Verification items for the finished model (mm, model axes). A direction names the side the tool comes from. Round coordinates to 2 decimals unless told otherwise and drop trailing zeros. Order: outer loops, then holes, each group sorted by start corner. A loop starts at its lowest first (then second) coordinate and runs counter-clockwise, first axis right, second up. Notation, with made-up numbers: (30, 46) -> (88, 46) arc R21 ccw to (88, 60) -> close; hole circle Ø8 at (-9.75, 41). An arc over 180 degrees is marked (long way). Put each result on its own line as item: value.
```python
from build123d import *

# Parameters (mm, degrees)
CROQUIS1_R              = 5.000000001
CROQUIS1_W              = 11.000000002
CROQUIS1_H              = 6.000000001
CROQUIS1_W_2            = 11.000000001
CROQUIS1_W_3            = 83.00000001
CROQUIS1_H_2            = 54.000000007
SALIENTE_EXTRUIR1_DEPTH = 1.5
CROQUIS3_W              = 3
CROQUIS3_H              = 143.999988457
SALIENTE_EXTRUIR2_DEPTH = 15
CROQUIS4_R              = 4.1
CORTAR_EXTRUIR1_DEPTH   = 23
CROQUIS8_W              = 20.699997559
CROQUIS8_H              = 3
SALIENTE_EXTRUIR4_DEPTH = 3
CROQUIS9_W              = 20.699997559
CROQUIS9_H              = 3
SALIENTE_EXTRUIR5_DEPTH = 3


with BuildPart() as part:
    # Croquis1 → Saliente-Extruir1 (new, symmetric)
    with BuildSketch(Plane.XY):
        Polygon((18.699888738, 146.999988499), (-0.000108821, 146.999988499), (-0.000108821, 3.000000042), (18.699888738, 3.000000042), (18.699888738, -1.1561e-05), (31.299897882, -1.1561e-05), (31.299897882, 2.999988439), (39.849897883, 2.999988439), (39.849897883, 6.5452e-05), (48.799897884, 6.5452e-05), (48.799897884, 3.000065452), (51.579549154, 3.000065452), (51.579549154, 6.749716476), (49.079130382, 6.749716476), (49.079130382, 9.750065453), (51.579549154, 9.750065453), (51.579549154, 10.725065453), (54.579549155, 10.725065453), (54.579549155, 9.750065453), (57.079549155, 9.750065453), (57.079549155, 6.749716476), (54.579549155, 6.749716476), (54.579549155, 3.000065452), (57.359200426, 3.000065452), (57.359200426, 9.8389e-05), (66.309200426, 9.8389e-05), (66.309200426, 3.00009839), (74.840541181, 3.00009839), (74.840541181, 9.8305e-05), (87.461202556, 0.000103657), (87.461202556, 3.000103699), (99.999885723, 3.000103699), (99.999885723, 9.999884868), (96.999885722, 9.999884868), (96.999885722, 19.999884869), (99.999885723, 19.999884869), (99.999885723, 29.99988487), (96.999885722, 29.99988487), (96.999885722, 43.437175485), (93.250234699, 43.437175485), (93.250234699, 40.937175485), (90.249885721, 40.937175485), (90.249885721, 43.437175485), (89.274885721, 43.437175485), (89.274885721, 46.437175486), (90.249885721, 46.437175486), (90.249885721, 48.937594258), (93.250234699, 48.937594258), (93.250234699, 46.437175486), (96.999885722, 46.437175486), (96.999885722, 59.874884873), (99.999885723, 59.874884873), (99.999885723, 69.999884875), (96.999885722, 69.999884875), (96.999885722, 79.999884876), (99.999885723, 79.999884876), (99.999885723, 90.124884877), (96.999885722, 90.124884877), (96.999885722, 103.562175492), (93.250234699, 103.562175492), (93.250234699, 101.062175492), (90.249885721, 101.062175492), (90.249885721, 103.562175492), (89.274885721, 103.562175492), (89.274885721, 106.562175493), (90.249885721, 106.562175493), (90.249885721, 109.062594265), (93.250234699, 109.062594265), (93.250234699, 106.562175493), (96.999885722, 106.562175493), (96.999885722, 119.99988488), (99.999885723, 119.99988488), (99.999885723, 129.999884881), (96.999885722, 129.999884881), (96.999885722, 139.999884883), (99.999885723, 139.999884883), (99.999885723, 146.999884842), (87.461202556, 146.999884842), (87.461202556, 149.999884884), (74.840541181, 149.999890236), (74.840541181, 146.999890151), (66.309200426, 146.999890151), (66.309200426, 149.999890151), (57.359200426, 149.999890151), (57.359200426, 146.999923088), (54.579549155, 146.999923088), (54.579549155, 143.250272065), (57.079549155, 143.250272065), (57.079549155, 140.249923087), (54.579549155, 140.249923087), (54.579549155, 139.274923087), (51.579549154, 139.274923087), (51.579549154, 140.249923087), (49.079130382, 140.249923087), (49.079130382, 143.250272065), (51.579549154, 143.250272065), (51.579549154, 146.999923088), (48.799897884, 146.999923088), (48.799897884, 149.999923089), (39.849897883, 149.999923089), (39.849897883, 147.000000101), (31.299897882, 147.000000101), (31.299897882, 150.000000101), (18.699888738, 150.000000101), align=None)
        with Locations((18.167765659, 72.011021453)):
            Circle(CROQUIS1_R, mode=Mode.SUBTRACT)
        with Locations((35.451849713, 72.011021453)):
            Rectangle(CROQUIS1_W, CROQUIS1_H, mode=Mode.SUBTRACT)
        with BuildLine():
            Line((82.774554778, 63.495021452), (82.774554778, 61.971021451))
            Line((82.774554778, 61.971021451), (85.314554779, 59.431021451))
            Line((85.314554779, 59.431021451), (85.314554779, 26.411021447))
            Line((85.314554779, 26.411021447), (82.774554778, 23.871021447))
            Line((82.774554778, 23.871021447), (82.774554778, 12.441021446))
            Line((82.774554778, 12.441021446), (81.504554778, 11.171021446))
            Line((81.504554778, 11.171021446), (17.750554771, 11.171021446))
            ThreePointArc((17.750554771, 11.171021446), (17.032134281, 11.468600956), (16.734554771, 12.187021446))
            Line((16.734554771, 12.187021446), (16.734554771, 63.495021452))
            ThreePointArc((16.734554771, 63.495021452), (17.032134281, 64.213441941), (17.750554771, 64.511021452))
            Line((17.750554771, 64.511021452), (81.758554778, 64.511021452))
            ThreePointArc((81.758554778, 64.511021452), (82.476975268, 64.213441941), (82.774554778, 63.495021452))
        make_face(mode=Mode.SUBTRACT)
        with Locations((57.631849716, 72.011021453)):
            Rectangle(CROQUIS1_W_2, CROQUIS1_H, mode=Mode.SUBTRACT)
        with Locations((79.814554778, 72.011021453)):
            Rectangle(CROQUIS1_W, CROQUIS1_H, mode=Mode.SUBTRACT)
        with Locations((45.799885716, 106.511021457)):
            Rectangle(CROQUIS1_W_3, CROQUIS1_H_2, mode=Mode.SUBTRACT)
        with Locations((15.358852485, 137.999884882)):
            Rectangle(CROQUIS1_W_2, CROQUIS1_H, mode=Mode.SUBTRACT)
        with Locations((41.342185821, 137.999884882)):
            Rectangle(CROQUIS1_W_2, CROQUIS1_H, mode=Mode.SUBTRACT)
        with Locations((65.074870839, 137.999884882)):
            Rectangle(CROQUIS1_W_2, CROQUIS1_H, mode=Mode.SUBTRACT)
        with Locations((85.358852493, 137.999884882)):
            Rectangle(CROQUIS1_W_2, CROQUIS1_H, mode=Mode.SUBTRACT)
    extrude(amount=SALIENTE_EXTRUIR1_DEPTH, both=True)

    # Croquis3 → Saliente-Extruir2 (add)
    with BuildSketch(Plane.ZY.offset(0.000108821)):
        with Locations((0, 74.999994271)):
            Rectangle(CROQUIS3_W, CROQUIS3_H)
    extrude(amount=SALIENTE_EXTRUIR2_DEPTH)

    # Croquis4 → Cortar-Extruir1 (cut)
    with BuildSketch(Plane.XY.offset(1.5)):
        with Locations((-7.499965561, 11.700000042)):
            Circle(CROQUIS4_R)
        with BuildLine():
            Line((-5.999990973, 127.200018373), (-8.499990973, 127.200018373))
            ThreePointArc((-8.499990973, 127.200018373), (-8.853544364, 127.053571764), (-8.999990973, 126.700018373))
            Line((-8.999990973, 126.700018373), (-8.999990973, 124.700000042))
            ThreePointArc((-8.999990973, 124.700000042), (-8.853544364, 124.346446651), (-8.499990973, 124.200000042))
            Line((-8.499990973, 124.200000042), (-5.999990973, 124.200000042))
            Line((-5.999990973, 124.200000042), (-5.999990973, 127.200018373))
        make_face()
    extrude(amount=-CORTAR_EXTRUIR1_DEPTH, mode=Mode.SUBTRACT)

    # Croquis8 → Saliente-Extruir4 (add)
    with BuildSketch(Plane.XZ.offset(-3.000000042)):
        with Locations((-4.650110042, 0)):
            Rectangle(CROQUIS8_W, CROQUIS8_H)
    extrude(amount=SALIENTE_EXTRUIR4_DEPTH)

    # Croquis9 → Saliente-Extruir5 (add)
    with BuildSketch(Plane(origin=(0, 146.999988499, 0), x_dir=(1, 0, 0), z_dir=(0, 1, 0))):
        with Locations((-4.650110042, 0)):
            Rectangle(CROQUIS9_W, CROQUIS9_H)
    extrude(amount=SALIENTE_EXTRUIR5_DEPTH)


solid = part.part
```
Item 1: Sectioned sample at B-B, the plane x = 27.5. Record the boundary of the cut face in (y, z), then the cut area to 3 significant figures.
Geometry check:
outline: (0, -1.5) -> (11.17, -1.5) -> (11.17, 1.5) -> (0, 1.5) -> close; (64.51, -1.5) -> (79.51, -1.5) -> (79.51, 1.5) -> (64.51, 1.5) -> close; (133.51, -1.5) -> (150, -1.5) -> (150, 1.5) -> (133.51, 1.5) -> close
area: 128 mm2
Item 2: Sectioned sample at C-C, the plane z = -0.45. Give the number of separate pieces and of enclosed holes in the cut face, then the cut area to 3 significant figures.
Geometry check:
separate pieces: 1
enclosed holes: 12
area: 7,830 mm2
Item 3: Tool access check on faces 1 (the face through (36, 3, 0)), 2 (the face through (87.461, 148, 0)), 3 (the face through (89.275, 105, 0)), 4 (the face through (57.08, 8, 0)), 5 (the face through (94, 3, 0)). Record the directions out of +Z, -Z, +X, -X, +Y, -Y that give a thin tool (end or side, any length) a straight path to the whole face; none if there is none.
Geometry check:
face 1: +Z, -Z, -Y
face 2: +Z, -Z, +X, +Y
face 3: +Z, -Z, +X
face 4: +Z, -Z
face 5: +Z, -Z, +X, -Y
Item 4: Sectioned sample at A-A, the plane y = 115. Record the boundary of the cut face in (x, z).
Geometry check:
outline: (-15, -1.5) -> (4.3, -1.5) -> (4.3, 1.5) -> (-15, 1.5) -> close; (87.3, -1.5) -> (97, -1.5) -> (97, 1.5) -> (87.3, 1.5) -> close
Item 5: Release check for a two-part mould opening along Y. For faces 6 (the face through (16.735, 37, 0)), 7 (the face through (81, 0, 0)), 8 (the face through (18.7, 2, 0)), 9 (the face through (49.079, 142, 0)) record: pulls with the +Y half, pulls with the -Y half, needs draft (parallel to the pull), parting line crosses it, or undercut.
Geometry check:
face 6: undercut
face 7: pulls with the -Y half
face 8: needs draft
face 9: undercut
Item 6: Depth check by flat-ended pin: pin 1 Ø0.8 at (x, z) = (90, 0.5) entering from -Y; pin 2 Ø1.5 at (y, z) = (105, 0) entering from +X; pin 3 Ø0.9 at (y, z) = (149, 0.5) entering from +X. Enter the tip coordinate at first touch or a pass-through.
Geometry check:
pin 1: y = 3
pin 2: x = 89.27
pin 3: x = 87.46
Item 7: Material ranges on line 1 along Y through (x, z) = (46, -0.85); line 2 along Y through (x, z) = (10.5, 1.2); line 3 along Y through (x, z) = (18, -1.4), recorded low to high.
Geometry check:
line 1: 0 to 11.17, 64.51 to 79.51, 133.51 to 135, 141 to 150
line 2: 3 to 79.51, 133.51 to 135, 141 to 147
line 3: 3 to 11.17, 64.51 to 67.01, 77.01 to 79.51, 133.51 to 135, 141 to 147
